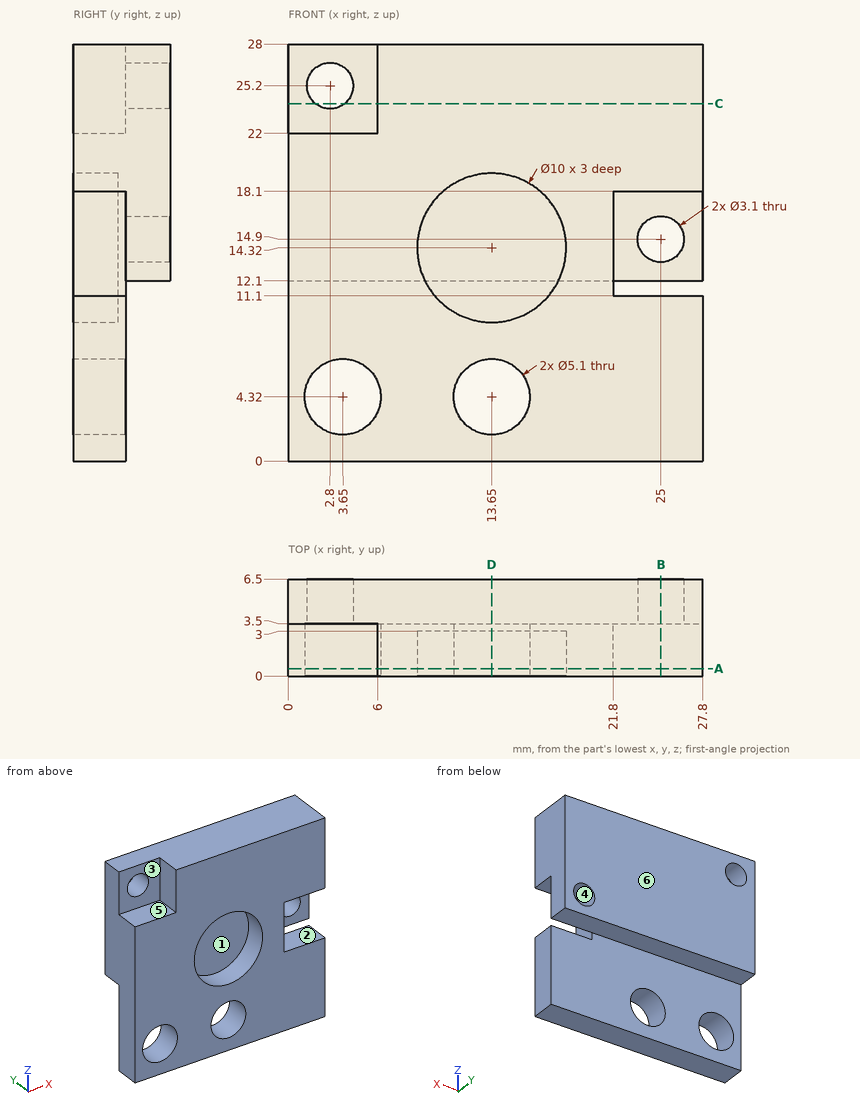
Geometry check sheet. Reference: drawing and pictorial views, mm from the part's lowest x, y, z. A direction names the side the tool comes from. Round coordinates to 2 decimals unless told otherwise and drop trailing zeros. Loops run counter-clockwise (first coordinate to the right, second up) from the corner with the lowest first, then second, coordinate; pieces in that order, holes last.
1. Sectioned sample at D-D on x = 13.65. Record the boundary of the cut face in (y, z).
2. Scan lines: probe 1 along Z at (x, y) = (23.75, 2.5); probe 2 along X at (y, z) = (1.5, 14.5); probe 3 along X at (y, z) = (5.5, 14.9). Record each from-to range of solid material in increasing order.
3. Mould release check, pull along Z, two halves, no side actions. Record for the marked faces 4, 5 and 6: released by +Z, released by -Z, zero draft, split by the parting line, or undercut.
4. Set-up check for the marked faces 1, 2 and 3: record each of +Z, -Z, +X, -X, +Y, -Y from which the full face is reachable in a straight line by a thin tool's end or side.
5. Sectioned sample at B-B on x = 25. Record the boundary of the cut face in (y, z).
6. Sectioned sample at C-C on z = 24. Record the boundary of the cut face in (x, y), and give its area (3 significant figures).
7. Gauge pin test, flat ends, axial feed: pin 1 Ø13.5 at (x, z) = (18.5, 7) entering from +Y; pin 2 Ø1.8 at (y, z) = (2, 24.5) entering from -X; pin 3 Ø4 at (x, z) = (3.65, 4.32) entering from +Y; pin 4 Ø3 at (x, z) = (16, 14) entering from -Y. Record the tip position at first contact, or that the pin passes through.
8. Sectioned sample at A-A on y = 0.5. Record the boundary of the cut face in (x, z), and give its area (3 significant figures).
Recorded:
1. outline: (0, 0) - (3.5, 0) - (3.5, 1.77) - (0, 1.77) - close; (0, 6.87) - (3.5, 6.87) - (3.5, 12.1) - (6.5, 12.1) - (6.5, 28) - (0, 28) - (0, 19.32) - (3, 19.32) - (3, 9.32) - (0, 9.32) - close
2. probe 1: z = 0 to 11.1, 18.1 to 28
2. probe 2: x = 0 to 8.65, 18.65 to 21.8
2. probe 3: x = 0 to 23.45, 26.55 to 27.8
3. face 4: undercut
3. face 5: released by +Z
3. face 6: zero draft
4. face 1: -Y
4. face 2: +X, +Y, -Y
4. face 3: +Z, -X, -Y
5. outline: (0, 0) - (3.5, 0) - (3.5, 11.1) - (0, 11.1) - close; (0, 18.1) - (3.5, 18.1) - (3.5, 16.45) - (6.5, 16.45) - (6.5, 28) - (0, 28) - close; (3.5, 12.1) - (6.5, 12.1) - (6.5, 13.35) - (3.5, 13.35) - close
6. outline: (0, 3.5) - (1.82, 3.5) - (1.82, 6.5) - (0, 6.5) - close; (3.78, 3.5) - (6, 3.5) - (6, 0) - (27.8, 0) - (27.8, 6.5) - (3.78, 6.5) - close
6. area: 154 mm2
7. pin 1: stops at y = 6.5
7. pin 2: stops at x = 6
7. pin 3: passes through
7. pin 4: stops at y = 3
8. outline: (0, 0) - (27.8, 0) - (27.8, 11.1) - (21.8, 11.1) - (21.8, 18.1) - (27.8, 18.1) - (27.8, 28) - (6, 28) - (6, 22) - (0, 22) - close; hole circle Ø5.1 at (3.65, 4.32); hole circle Ø10 at (13.65, 14.32); hole circle Ø5.1 at (13.65, 4.32)
8. area: 581 mm2
